from build123d import *

# Parameters (mm, degrees)
F0_R     = 14.5
F1_DEPTH = 3
F2_R     = 8.75
F3_DEPTH = 8
F4_R     = 1
F5_R     = 14.5
F5_R_2   = 12.75
F6_DEPTH = 5
F7_R     = 0.8


with BuildPart() as f1:
    # F0 (on Top) → F1 (new body)
    with BuildSketch(Plane.XY):
        Circle(F0_R)
    extrude(amount=F1_DEPTH)

    # F2 (on face) → F3 (join)
    with BuildSketch(Plane.XY.offset(3)):
        Circle(F2_R)
    extrude(amount=F3_DEPTH)

    # F4
    f4_edges = [f1.edges().sort_by_distance(p)[0] for p in [
        (-14.5, 0, 0),
    ]]
    fillet(f4_edges, radius=F4_R)

    # F5 (on face) → F6 (join)
    with BuildSketch(Plane.XY.offset(3)):
        Circle(F5_R)
        Circle(F5_R_2, mode=Mode.SUBTRACT)
    extrude(amount=F6_DEPTH)

    # F7
    f7_edges = [f1.edges().sort_by_distance(p)[0] for p in [
        (-14.5, 0, 8),
        (-12.75, 0, 8),
    ]]
    fillet(f7_edges, radius=F7_R)


solid = f1.part
For this review, take the finished solid that the model builds, in its own axes (mm). A direction names the side the tool comes from. Round coordinates to 2 decimals unless told otherwise and drop trailing zeros. Order: outer loops, then holes, each group sorted by start corner. A loop starts at its lowest first (then second) coordinate and runs counter-clockwise, first axis right, second up. Notation, with made-up numbers: M 12,-9.5 L 71,-9.5 A30 ccw 71,23.5 Z; hole C 23,65.5 d6. An arc over 180 degrees is marked long. Write each question's results on one line, items separated by ' | '. Start each with the question number.
1. Draft analysis for pull direction X (two halves, no side actions). For faces 1 (the face through (6.691, -12.864, 4.057)), 2 (the face through (0, 0, 0)), 3 (the face through (-6.944, -5.324, 6.944)), 4 (the face through (-9, -3, 3)), state which applies: pulls with the +X half, pulls with the -X half, needs draft (parallel to the pull), parting line crosses it, or undercut.
2. Tool access review of faces 5 (the face through (0, 0, 11)), 6 (the face through (-2.764, -12.447, 5.071)): name each direction out of +Z, -Z, +X, -X, +Y, -Y from which nothing blocks a thin tool from reaching the whole face with its end or side.
3. Clearance check with flat-ended pins moving along their axes: pin 1 Ø4 at (x, z) = (7, 4.5) entering from +Y; pin 2 Ø1 at (y, z) = (5.5, 5.5) entering from +X; pin 3 Ø3 at (y, z) = (11, 8.5) entering from -X. State where each tip first meets the part, or that it passes through.
4. Add section D-D (z = 9.5). State the section outline as (x, y) points.
5. Add section A-A (z = 4.75). State the section outline as (x, y) points, then the cut area to 3 significant figures.
6. Add section B-B (y = 0). State the section outline as (x, z) points, then the cut area to 3 significant figures.
7. To check wall thickness, follow L1, parallel to Y at x = 0, z = 5.35; L2, parallel to Y at x = -8, z = 4.5; L3, parallel to X at y = 2, z = 6.5. State the ranges of each line that lie inside material, in increasing order. Write a range as [from, to].
Output values:
1) face 1: parting line crosses it | face 2: needs draft | face 3: undercut | face 4: undercut
2) face 5: +Z, +X, -X, +Y, -Y | face 6: +Z
3) pin 1: y = 13.61 | pin 2: x = 13.61 | pin 3: x = -10.54
4) outline: C 0,0 d17.5
5) outline: C 0,0 d29; C 0,0 d17.5; hole C 0,0 d25.5 | area: 390 mm^2
6) outline: M -14.5,1 A1 ccw -13.5,0 L 13.5,0 A1 ccw 14.5,1 L 14.5,7.2 A0.8 ccw 13.7,8 L 13.55,8 A0.8 ccw 12.75,7.2 L 12.75,3 L 8.75,3 L 8.75,11 L -8.75,11 L -8.75,3 L -12.75,3 L -12.75,7.2 A0.8 ccw -13.55,8 L -13.7,8 A0.8 ccw -14.5,7.2 Z | area: 244 mm^2
7) L1: [-14.5, -12.75], [-8.75, 8.75], [12.75, 14.5] | L2: [-12.09, -9.93], [-3.54, 3.54], [9.93, 12.09] | L3: [-14.36, -12.59], [-8.52, 8.52], [12.59, 14.36]
